Read the model definition and answer for the solid it produces. Units are mm, in the model's axes. Give positions to 0.01 mm unless a question says otherwise; leave off trailing zeros. Loops run counter-clockwise (first coordinate to the right, second up) from the corner with the lowest first, then second, coordinate; pieces in that order, holes last.
(1) Find section B-B, the plane z = -39.96. Write down the section's boundary in (x, y), then the cut area to 3 significant figures.
(2) Straight lines are drawn through the part: probe 1 along Z at (x, y) = (-3.69, -0.4) (3 decimals); probe 2 along X at (y, z) = (-0.35, -36); probe 3 along Z at (x, y) = (-16.5, -1). For each, find the intervals that lie inside material, in ascending order.
(3) Each of these flat-tipped pins is pushed along its axis until it touches: P1, Ø1.7, axis at x = -3.69, z = -17.595, coming from the -Y side; P2, Ø3.5, axis at x = 48.55, z = -10.07, coming from the -Y side. Where does it stop, or does it pass through?
(4) Find section A-A, the plane x = -18.79. Write down the section's boundary in (y, z) (3 decimals), then the cut area to 3 significant figures.
(5) Find section C-C, the plane y = -0.6. State how many separate pieces and enclosed holes the cut face has, then the cut area to 3 significant figures.
(6) Find section D-D, the plane x = 7.5. Write down the section's boundary in (y, z), then the cut area to 3 significant figures.
Autodesk Inventor part; units mm, degrees
ref_plane "YZ Plane" through (0, 0, 0) normal (1, 0, 0) x (0, 1, 0)
ref_plane "XZ Plane" through (0, 0, 0) normal (0, 1, 0) x (-1, 0, 0)
ref_plane "XY Plane" through (0, 0, 0) normal (0, 0, 1) x (1, 0, 0)
sketch "Sketch1" plane through (0, 0, 0) normal (0, 1, 0) x (-1, 0, 0)
  line L0 (-44.2289, 0) -> (-44.2289, -28.14)
  line L1 (-0.4496, -28.14) -> (-0.4496, 0)
  circle A0 centre (-37.3393, -39.96) radius 1.55
  circle A1 centre (-22.3393, -39.96) radius 1.55
  circle A2 centre (-7.3393, -39.96) radius 1.55
  circle A3 centre (-48.5486, -10.07) radius 1.05
  circle A4 centre (-55.8486, -17.07) radius 1.05
  circle A5 centre (-55.8486, -3.07) radius 1.05
  circle A6 centre (-69.0686, -18.07) radius 1.05
  circle A7 centre (-69.0686, -2.07) radius 1.05
  circle A8 centre (18.79, -17.595) radius 1.05
  circle A9 centre (18.79, -2.545) radius 1.05
  circle A10 centre (3.69, -17.595) radius 1.05
  circle A11 centre (3.69, -2.545) radius 1.05
  arc A12 (30.49, -1) -> (29.49, 0) centre (29.49, -1) ccw
  line L2 (30.49, -1) -> (30.49, -4.1236)
  arc A13 (29.49, -28.14) -> (30.49, -27.14) centre (29.49, -27.14) ccw
  line L3 (29.49, -28.14) -> (-0.8993, -28.14)
  arc A14 (-75.1686, -27.14) -> (-74.1686, -28.14) centre (-74.1686, -27.14) ccw
  line L4 (-75.1686, -27.14) -> (-75.1686, -16.0164)
  line L5 (-43.7793, -28.14) -> (-74.1686, -28.14)
  line L6 (-43.7793, -50) -> (-43.7793, -28.14)
  line L7 (-0.8993, -50) -> (-43.7793, -50)
  line L8 (-0.8993, -28.14) -> (-0.8993, -50)
  line L9 (30.49, -16.0164) -> (30.49, -27.14)
  arc A15 (30.49, -4.1236) -> (30.49, -16.0164) centre (31.29, -10.07) ccw
  line L10 (-74.1686, 0) -> (29.49, 0)
  arc A16 (-74.1686, 0) -> (-75.1686, -1) centre (-74.1686, -1) ccw
  line L11 (-75.1686, -4.1236) -> (-75.1686, -1)
  arc A17 (-75.1686, -16.0164) -> (-75.1686, -4.1236) centre (-75.9686, -10.07) ccw
  line L12 (-44.6786, -28.14) -> (-44.6786, 0)
  line L13 (-43.7793, 0) -> (-43.7793, -28.14)
  line L14 (-0.8993, -28.14) -> (-0.8993, 0)
  line L15 (0, 0) -> (0, -28.14)
extrude "Extrusion1" add sketch "Sketch1" against normal blind 1.5
properties part number "axis_23_top_frame"
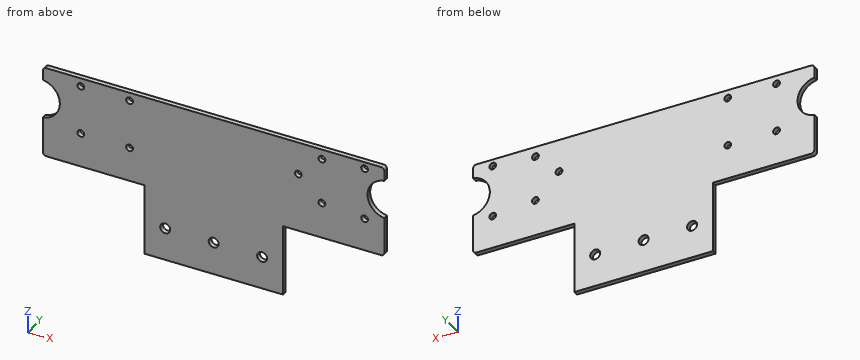
Entries:
1. outline: (0.9, -1.5) - (5.79, -1.5) - (5.79, 0) - (0.9, 0) - close; (8.89, -1.5) - (20.79, -1.5) - (20.79, 0) - (8.89, 0) - close; (23.89, -1.5) - (35.79, -1.5) - (35.79, 0) - (23.89, 0) - close; (38.89, -1.5) - (43.78, -1.5) - (43.78, 0) - (38.89, 0) - close
1. area: 50.4 mm2
2. probe 1: z = -28.14 to -18.645, -16.545 to -3.595, -1.495 to 0
2. probe 2: x = 0.9 to 43.78
2. probe 3: z = -28.14 to 0
3. P1: passes through
3. P2: stops at y = -1.5
4. outline: (-1.5, -28.14) - (0, -28.14) - (0, -18.645) - (-1.5, -18.645) - close; (-1.5, -16.545) - (0, -16.545) - (0, -3.595) - (-1.5, -3.595) - close; (-1.5, -1.495) - (0, -1.495) - (0, 0) - (-1.5, 0) - close
4. area: 35.9 mm2
5. separate pieces: 1
5. enclosed holes: 12
5. area: 3,760 mm2
6. outline: (-1.5, -50) - (0, -50) - (0, -41.5) - (-1.5, -41.5) - close; (-1.5, -38.42) - (0, -38.42) - (0, 0) - (-1.5, 0) - close
6. area: 70.4 mm2
